Can you work these out from the model? Positions are in its coordinate system, mm. Give positions to 0.01 mm unless a question says otherwise; leave off trailing zeros. Order: outer loops, then holes, each group sorted by start corner. A loop starts at its lowest first (then second) coordinate and runs counter-clockwise, first axis right, second up.
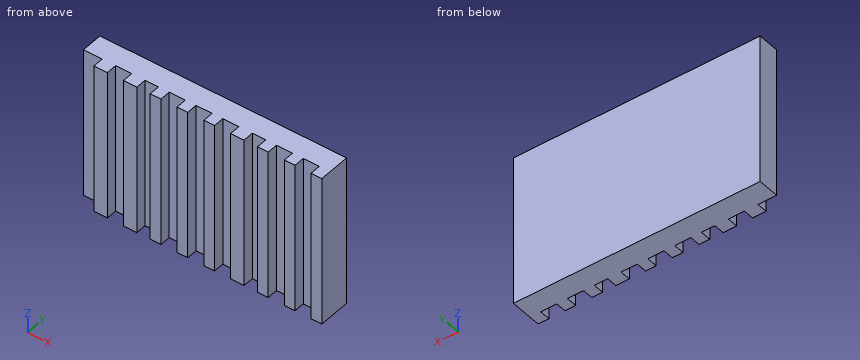
```python
from build123d import *

# Parameters (mm, degrees)
BOSS_EXTRUDE1_DEPTH = 28


with BuildPart() as part:
    # Sketch1 → Boss-Extrude1 (new body)
    with BuildSketch(Plane.XY):
        Polygon((-23, -1.000000551), (-19.500008127, -1.000000551), (-19.500008127, -3), (-17.000007621, -3), (-17.000007621, -1.000000551), (-14.000005953, -1.000000551), (-14.000005953, -3), (-11.500005447, -3), (-11.500005447, -1.000000551), (-9.000004942, -1.000000551), (-9.000004942, -3), (-7.000005493, -3), (-7.000005493, -1.000000551), (-4.000003825, -1.000000551), (-4.000003825, -3), (-2.000004376, -3), (-2.000004376, -1.000000551), (0.999997292, -1.000000551), (0.999997292, -3), (2.99999674, -3), (2.99999674, -1.000000551), (5.999998408, -1.000000551), (5.999998408, -3), (8.499998914, -3), (8.499998914, -1.000000551), (10.99999942, -1.000000551), (10.99999942, -3), (12.999998868, -3), (12.999998868, -1.000000551), (16.000000536, -1.000000551), (16.000000536, -3), (17.999999985, -3), (17.999999985, -1.000000551), (21.000001653, -1.000000551), (21.000001653, -3), (23.000001102, -3), (23.000001102, 3), (-23, 3), align=None)
    extrude(amount=BOSS_EXTRUDE1_DEPTH)


solid = part.part
```
1) Suppose I cut it at B-B (x = -16.5). Please give me the cut outline in (y, z), and give its area (3 significant figures).
2) If I drill on line 1 (Y direction, x = 15.5, z = 24), over which ranges is the centre line in solid material (lowest first)?
3) I'm going to push flat-ended pins straight in: pin 1 Ø0.9 at (x, z) = (-16, 10) entering from -Y; pin 2 Ø1.6 at (y, z) = (-2.5, 18) entering from -X. Where does each tip first touch, or does it pass through?
4) Suppose I cut it at A-A (y = -2.3). Give the number of separate pieces and of enclosed holes in the cut face, and give its area (3 significant figures).
Results:
1. outline: (-1, 0) - (3, 0) - (3, 28) - (-1, 28) - close
1. area: 112 mm2
2. line 1: y = -1 to 3
3. pin 1: stops at y = -1
3. pin 2: stops at x = -19.5
4. separate pieces: 9
4. enclosed holes: 0
4. area: 546 mm2
